Source: CAD feature listing. Evaluate the final solid. Frame: model axes, mm. A direction names the side the tool comes from. Coordinates: 2 decimals unless noted, no trailing zeros. Loops run counter-clockwise (first coordinate to the right, second up) from the corner with the lowest first, then second, coordinate; pieces in that order, holes last.
```python
from build123d import *

# Parameters (mm, degrees)
F0_R     = 1.6
F1_DEPTH = 1.75
F2_W     = 7.2
F2_H     = 12
F2_W_2   = 9
F3_DEPTH = 12
F4_W     = 12
F4_H     = 9
F4_W_2   = 2
F5_DEPTH = 11
F6_W     = 21
F6_H     = 3
F6_W_2   = 16
F6_W_3   = 25.5
F7_DEPTH = 8


with BuildPart() as f1:
    # F0 (on Top) → F1 (new body)
    with BuildSketch(Plane.XY):
        Polygon((29.560432, 36.989467), (-36.439568, 36.989467), (-36.439568, -16.010533), (29.560432, -16.010533), (29.560432, -13.644766), (32.560432, -10.644766), (32.560432, 21.065632), (29.560432, 24.065632), align=None)
        with Locations((-22.939568, -13.510533)):
            Circle(F0_R, mode=Mode.SUBTRACT)
        with Locations((29.860432, -8.510533)):
            Circle(F0_R, mode=Mode.SUBTRACT)
        with Locations((-20.939568, 34.489467)):
            Circle(F0_R, mode=Mode.SUBTRACT)
        with Locations((29.860432, 19.489467)):
            Circle(F0_R, mode=Mode.SUBTRACT)
    extrude(amount=F1_DEPTH)

    # F2 (on face) → F3 (join)
    with BuildSketch(Plane.XY.offset(1.75)):
        with Locations((-40.039568, 21.989467)):
            Rectangle(F2_W, F2_H)
        with Locations((-31.939568, 21.989467)):
            Rectangle(F2_W_2, F2_H)
    extrude(amount=F3_DEPTH)

    # F4 (on face) → F5 (join)
    with BuildSketch(Plane.XY.offset(1.75)):
        with Locations((-30.439568, -7.510533)):
            Rectangle(F4_W, F4_H)
        with Locations((-37.439568, -7.510533)):
            Rectangle(F4_W_2, F4_H)
    extrude(amount=F5_DEPTH)

    # F6 (on face) → F7 (join)
    with BuildSketch(Plane.XY.offset(1.75)):
        with Locations((1.060432, -13.510533)):
            Rectangle(F6_W, F6_H)
        with Locations((20.560432, -13.510533)):
            Rectangle(F6_W_2, F6_H)
        with Locations((18.060432, 34.489467)):
            Rectangle(F6_W, F6_H)
        with Locations((-6.189568, 34.489467)):
            Rectangle(F6_W_3, F6_H)
    extrude(amount=F7_DEPTH)


solid = f1.part
```
Q1. Reachability of faces 1 (the flat face through (29.56, 30, 1)), 2 (the flat face through (-36.44, 11, 1)), 3 (the flat face through (-9.44, -14, 6)) from +Z, -Z, +X, -X, +Y, -Y: full face, straight path, thin tool, end or side. Return the list, or none.
Q2. Material intervals for line 1 along Y through (x, z) = (2.5, 3); line 2 along X through (y, z) = (-13, 2.5); line 3 along Y through (x, z) = (-34, 4.75), sorted ascending.
Q3. Section query A-A on z = 11.75. Return the cut outline in (x, y).
Q4. Section query B-B on x = -30. Return the cut outline in (y, z), then the cut area to 3 significant figures.
Q5. First-contact query: pin 1 Ø6 at (x, z) = (-32.5, 6.5) entering from -Y; pin 2 Ø6 at (x, z) = (-14, 5.5) entering from +Y; pin 3 Ø2 at (y, z) = (16.5, 11.5) entering from +X. Flat tips, straight axial feed; report the tip coordinate or a pass-through.
Q6. Draft query along Y for faces 4 (the flat face through (31.081, 22.545, 0.863)), 5 (the flat face through (-6, 32.989, 6)), 6 (the flat face through (20, -12.011, 6)), 7 (the flat face through (-37, -7, 1.75)). Return one class per face: released by +Y, released by -Y, zero draft, split by the parting line, or undercut.
Q7. Section query D-D on y = 30. Return the cut outline in (x, z).
Q8. Section query C-C on z = 7.75. Return the cut outline in (x, y).
Resolved:
1. face 1: +Z, -Z, +X, +Y
1. face 2: -Z, -X, +Y, -Y
1. face 3: +Z, -X, -Y
2. line 1: y = -15.01 to -12.01, 32.99 to 35.99
2. line 2: x = -9.44 to 11.56, 12.56 to 28.56
2. line 3: y = -12.01 to -3.01, 15.99 to 27.99
3. outline: (-43.64, 15.99) - (-27.44, 15.99) - (-27.44, 27.99) - (-43.64, 27.99) - close; (-38.44, -12.01) - (-24.44, -12.01) - (-24.44, -3.01) - (-38.44, -3.01) - close
4. outline: (-16.01, 0) - (36.99, 0) - (36.99, 1.75) - (27.99, 1.75) - (27.99, 13.75) - (15.99, 13.75) - (15.99, 1.75) - (-3.01, 1.75) - (-3.01, 12.75) - (-12.01, 12.75) - (-12.01, 1.75) - (-16.01, 1.75) - close
4. area: 336 mm2
5. pin 1: stops at y = -12.01
5. pin 2: stops at y = 35.99
5. pin 3: stops at x = -27.44
6. face 4: released by +Y
6. face 5: undercut
6. face 6: undercut
6. face 7: zero draft
7. outline: (-36.44, 0) - (29.56, 0) - (29.56, 1.75) - (-36.44, 1.75) - close
8. outline: (-43.64, 15.99) - (-27.44, 15.99) - (-27.44, 27.99) - (-43.64, 27.99) - close; (-38.44, -12.01) - (-24.44, -12.01) - (-24.44, -3.01) - (-38.44, -3.01) - close; (-18.94, 32.99) - (6.56, 32.99) - (6.56, 35.99) - (-18.94, 35.99) - close; (-9.44, -15.01) - (11.56, -15.01) - (11.56, -12.01) - (-9.44, -12.01) - close; (7.56, 32.99) - (28.56, 32.99) - (28.56, 35.99) - (7.56, 35.99) - close; (12.56, -15.01) - (28.56, -15.01) - (28.56, -12.01) - (12.56, -12.01) - close
